Part print with two shaded views. Sizes in mm from the minimum x, y, z corner. Coordinates: 2 decimals unless noted, no trailing zeros. Order: outer loops, then holes, each group sorted by start corner. A loop starts at its lowest first (then second) coordinate and runs counter-clockwise, first axis right, second up.
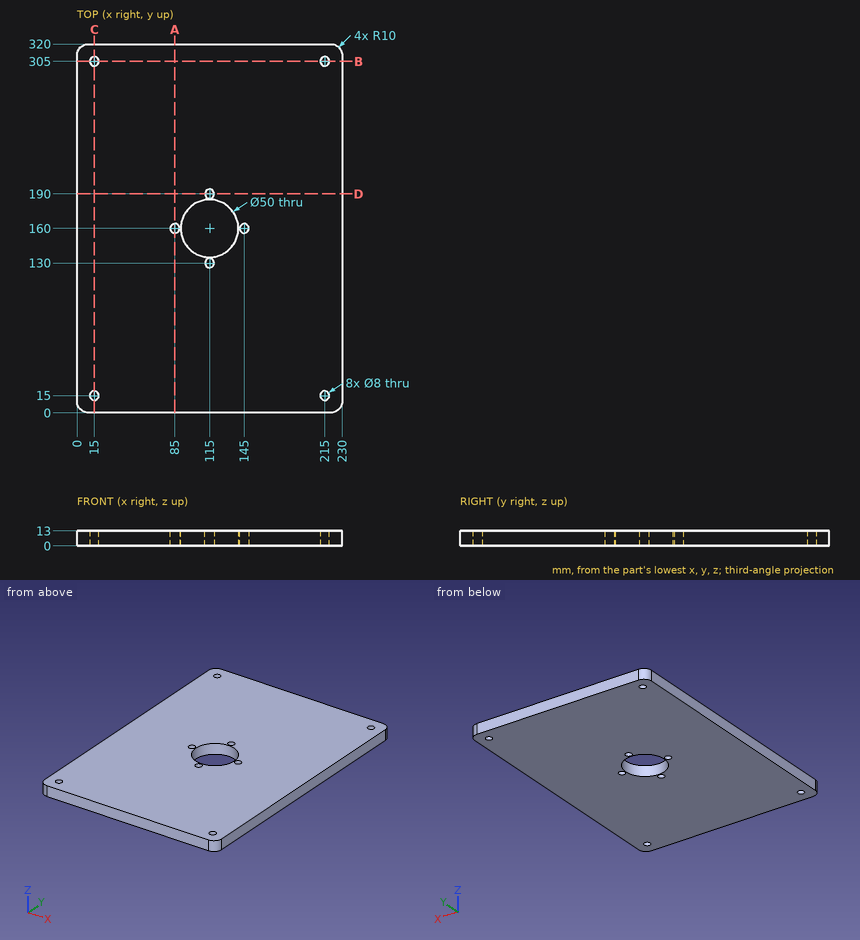
Q1. Pin check, flat tip, straight feed: pin 1 Ø7 at (x, y) = (215, 15) entering from -Z. Stop position of the tip, or through.
Results list:
pin 1: passes through
Q2. Cut at D-D on y = 190. Write the cut outline in (x, z), and give its area (3 significant figures).
Results list:
outline: (0, 0) - (111, 0) - (111, 13) - (0, 13) - close; (119, 0) - (230, 0) - (230, 13) - (119, 13) - close
area: 2,890 mm2
Q3. Cut at B-B on y = 305. Write the cut outline in (x, z).
Results list:
outline: (0, 0) - (11, 0) - (11, 13) - (0, 13) - close; (19, 0) - (211, 0) - (211, 13) - (19, 13) - close; (219, 0) - (230, 0) - (230, 13) - (219, 13) - close
Q4. Cut at C-C on x = 15. Write the cut outline in (y, z), and give its area (3 significant figures).
Results list:
outline: (0, 0) - (11, 0) - (11, 13) - (0, 13) - close; (19, 0) - (301, 0) - (301, 13) - (19, 13) - close; (309, 0) - (320, 0) - (320, 13) - (309, 13) - close
area: 3,950 mm2
Q5. Cut at A-A on x = 85. Write the cut outline in (y, z), and give its area (3 significant figures).
Results list:
outline: (0, 0) - (156, 0) - (156, 13) - (0, 13) - close; (164, 0) - (320, 0) - (320, 13) - (164, 13) - close
area: 4,060 mm2
Q6. Wall check: line 1 along Y through (x, z) = (115, 9.5); line 2 along X through (y, z) = (305, 7.5); line 3 along Y through (x, z) = (15, 5.5). Give the ranges that are in metal, low to high.
Results list:
line 1: y = 0 to 126, 134 to 135, 185 to 186, 194 to 320
line 2: x = 0 to 11, 19 to 211, 219 to 230
line 3: y = 0 to 11, 19 to 301, 309 to 320
